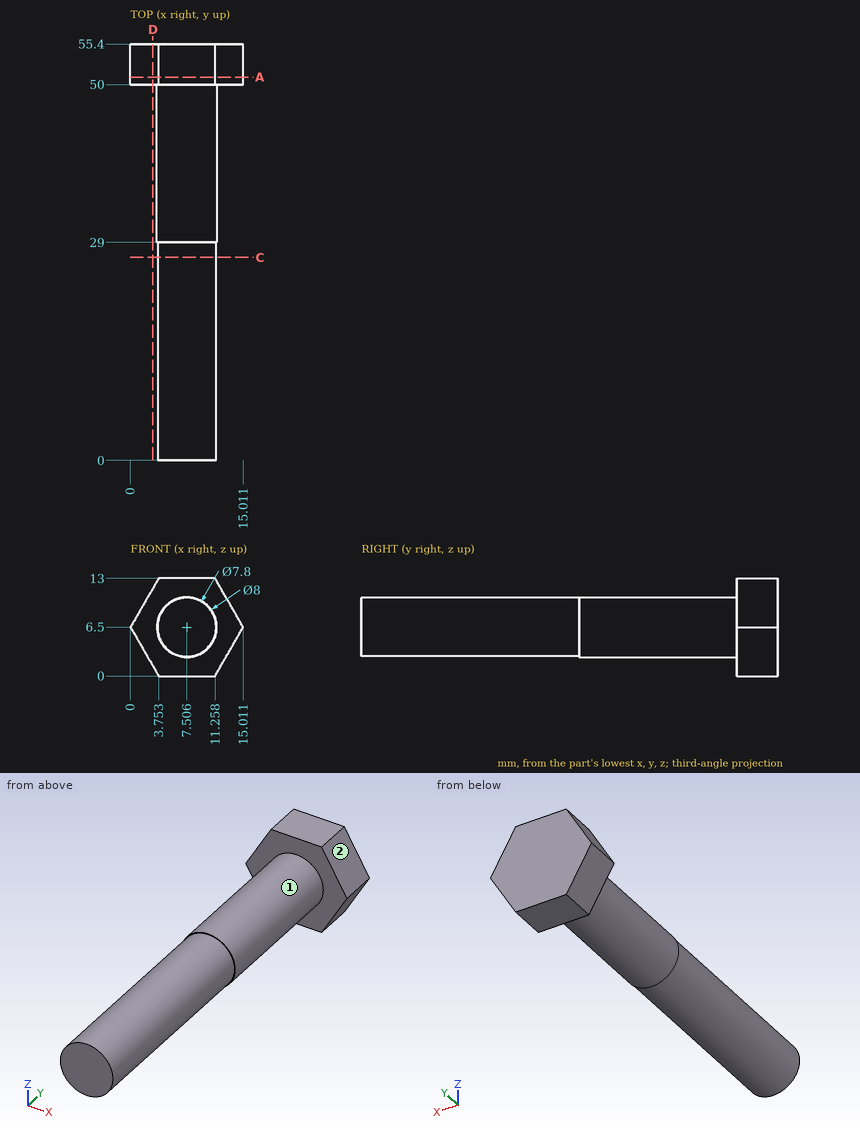
Could you check a few things on this drawing? It's one solid part, dimensions in mm from its lowest x, y, z. A direction names the side the tool comes from. Coordinates: 2 decimals unless noted, no trailing zeros. Order: outer loops, then holes, each group sorted by start corner. A loop starts at its lowest first (then second) coordinate and runs counter-clockwise, first axis right, second up. Notation, with made-up numbers: M -6.5,21.5 L 14.5,21.5 A11 ccw 14.5,40.5 Z; hole C 6.5,86.5 d7. An arc over 180 degrees is marked long. Answer as CSV lines item,"result".
(1) On a 3-axis mill with a long thin cutter (end or side, diameter ignored), from which of +Z, -Z, +X, -X, +Y, -Y can I reach the whole of each face in a straight line? I mean the marked faces 1 and 2. Say none if no direction works.
Geometry check:
face 1,"-Y"
face 2,"+Z, +X, +Y, -Y"
(2) Please list where these lines run through material, in increasing order: L1, parallel to Y at x = 4, z = 12.25; L2, parallel to Z at x = 7.25, y = 45; L3, parallel to X at y = 52, z = 11.25.
Geometry check:
L1,"50 to 55.4"
L2,"2.51 to 10.49"
L3,"2.74 to 12.27"
(3) I'm going to push flat-ended pins straight in: pin 1 (1.5 mm diameter, centred on x = 12.5, y = 41, fed in from +Z); pin 2 (4 mm diameter, centred on x = 5.5, y = 30, fed in from +Z). Where does each tip first touch, or does it pass through?
Geometry check:
pin 1,"through"
pin 2,"z = 10.5"
(4) Suppose I cut it at A-A on y = 51. Please give me the cut outline in (x, z).
Geometry check:
outline,"M 0,6.5 L 3.75,0 L 11.26,0 L 15.01,6.5 L 11.26,13 L 3.75,13 Z"
(5) Suppose I cut it at D-D on x = 3. Please give me the cut outline in (y, z).
Geometry check:
outline,"M 50,1.3 L 55.4,1.3 L 55.4,11.7 L 50,11.7 Z"
(6) Suppose I cut it at C-C on y = 27. Please give me the cut outline in (x, z) (1 decimal), plus the area to 3 significant figures.
Geometry check:
outline,"C 7.5,6.5 d7.8"
area,"47.8 mm^2"
